Input: part model. Units: mm. Frame: model coordinates. Face numbers are marked on the shaded views. A direction names the side the tool comes from. Coordinates: 2 decimals unless noted, no trailing zeros. Write each loop counter-clockwise with the first axis right and the second up, starting at its lowest first coordinate (ties: lowest second). Pieces come first, ordered by that corner, then holes. Notation, with made-up numbers: (6, 48) - (53, 48) arc R32 ccw to (53, 74) - close; hole circle Ø7 at (28.5, 57.25). An arc over 180 degrees is marked (long way). Use a Markdown table: item, result. Add a question column.
Q1. Section query D-D (z = 16.75). Return the cut outline in (x, y), then the cut area to 3 significant figures.
Q2. Pin query (flat end, axial travel): P1, Ø6, axis at x = 5, z = 15, coming from the +Y side; P2, Ø10, axis at x = -6, z = 12.5, coming from the +Y side; P3, Ø3, axis at y = 2.5, z = 8, coming from the -X side. Return the tip coordinate at first contact, or that it passes through.
Q3. Mould query, pull axis Z, two halves, no side actions, for the marked faces 1, 2, 3 and 4. Classes: released by +Z, released by -Z, zero draft, split by the parting line, or undercut.
Q4. Section query B-B (z = 5). Return the cut outline in (x, y).
Q5. Section query A-A (z = 11). Return the cut outline in (x, y).
Q6. Material intervals for probe 1 along Z at (x, y) = (8.5, 10); probe 2 along X at (y, z) = (-3, 6.5); probe 3 along Y at (x, z) = (2, 12), sorted ascending. Write a range as from..to.
Q7. Section query C-C (z = 2.25). Return the cut outline in (x, y).
Q8. Set-up query: the marked faces 5, 6 and 7. Return all of +Z, -Z, +X, -X, +Y, -Y with unobstructed straight access to the full face (end or side cutting, diameter ignored); none if empty.
from build123d import *

# Parameters (mm, degrees)
ESQUISSE1_W             = 5
ESQUISSE1_H             = 4.088235294
BOSS_EXTRU_1_DEPTH      = 20
ENL_V_START             = -16
ENL_V_MAT_EXTRU_1_DEPTH = 12
CHANFREIN1_SIZE         = 3
ESQUISSE3_R             = 2
ENL_V_MAT_EXTRU_2_DEPTH = 12
ENL_V_START_2           = -8
ESQUISSE4_R             = 4
ENL_V_MAT_EXTRU_3_DEPTH = 12


with BuildPart() as part:
    # Esquisse1 → Boss.-Extru.1 (new body)
    with BuildSketch(Plane.XY):
        with BuildLine():
            ThreePointArc((-14.409025375, 0), (1.090974625, 15.5), (16.590974625, 0))
            Line((16.590974625, 0), (11.590974625, 0))
            Line((11.590974625, 0), (-9.409025375, 0))
            Line((-9.409025375, 0), (-14.409025375, 0))
        make_face()
        with Locations((-11.909025375, -2.044117647)):
            Rectangle(ESQUISSE1_W, ESQUISSE1_H)
        with Locations((14.090974625, -2.044117647)):
            Rectangle(ESQUISSE1_W, ESQUISSE1_H)
    extrude(amount=BOSS_EXTRU_1_DEPTH)

    # Esquisse2 → Enlèv. mat.-Extru.1 (cut)
    with BuildSketch(Plane.XY.offset(20).offset(ENL_V_START)):
        with BuildLine():
            ThreePointArc((-14.409025375, 0), (1.090974625, 11.286497475), (16.590974625, 0))
            ThreePointArc((16.590974625, 0), (1.090974625, 15.5), (-14.409025375, 0))
        make_face()
    extrude(amount=ENL_V_MAT_EXTRU_1_DEPTH, mode=Mode.SUBTRACT)

    # Chanfrein1
    # the kernel refuses this chamfer: 3 mm, written as the material it takes off along each edge
    with BuildSketch(Plane(origin=(1.090974625, 0, 4), x_dir=(0.8782789278300123, -0.4781486431328276, 0), z_dir=(-0.4781486431328276, -0.8782789278300123, 0))) as chanfrein1_piece_1_section:
        Polygon((15.5, -CHANFREIN1_SIZE), (15.5 - CHANFREIN1_SIZE, 0), (15.5, 0), align=None)
    chanfrein1_piece_1 = revolve(axis=Axis((1.090974625, 0, 4), (0, 0, 1)), revolution_arc=237.129113272, mode=Mode.PRIVATE)
    chanfrein1_piece_1 = chanfrein1_piece_1 - Plane(origin=(1.090974625, -5, 2.541086631), x_dir=(-0.9517086177605509, 0.3070027799227584, 0), z_dir=(0, 0, -1)) * Cylinder(16.286497475, 63, mode=Mode.PRIVATE)
    add(chanfrein1_piece_1, mode=Mode.SUBTRACT)
    with BuildSketch(Plane(origin=(1.090974625, 0, 16), x_dir=(0.8782789278300122, -0.4781486431328277, 0), z_dir=(-0.4781486431328277, -0.8782789278300122, 0))) as chanfrein1_piece_2_section:
        Polygon((15.5, CHANFREIN1_SIZE), (15.5 - CHANFREIN1_SIZE, 0), (15.5, 0), align=None)
    chanfrein1_piece_2 = revolve(axis=Axis((1.090974625, 0, 16), (0, 0, 1)), revolution_arc=237.129113272, mode=Mode.PRIVATE)
    chanfrein1_piece_2 = chanfrein1_piece_2 - Plane(origin=(1.090974625, -5, 17.458913369), x_dir=(-0.9517086177605509, 0.3070027799227584, 0), z_dir=(0, 0, -1)) * Cylinder(16.286497475, 62, mode=Mode.PRIVATE)
    add(chanfrein1_piece_2, mode=Mode.SUBTRACT)

    # Esquisse3 → Enlèv. mat.-Extru.2 (cut)
    with BuildSketch(Plane.XZ):
        with Locations(Location((1.090974625, 10, 0), (0, 0, 270))):
            Circle(ESQUISSE3_R)
    extrude(amount=-ENL_V_MAT_EXTRU_2_DEPTH, mode=Mode.SUBTRACT)

    # Esquisse4 → Enlèv. mat.-Extru.3 (cut)
    with BuildSketch(Plane.XZ.offset(ENL_V_START_2)):
        with Locations(Location((1.090974625, 10, 0), (0, 0, 270))):
            Circle(ESQUISSE4_R)
    extrude(amount=-ENL_V_MAT_EXTRU_3_DEPTH, mode=Mode.SUBTRACT)


solid = part.part
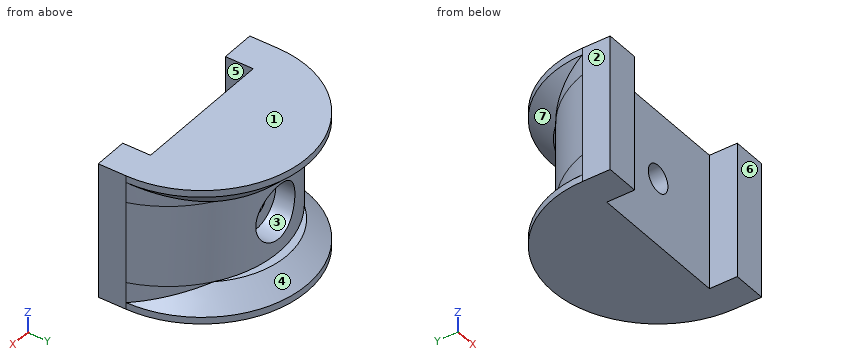
Values follow:
| question | item | result |
|---|---|---|
| 1 | outline | (-14.41, -4.09) - (-9.41, -4.09) - (-9.41, 0) - (11.59, 0) - (11.59, -4.09) - (16.59, -4.09) - (16.59, 0) arc R16.29 ccw to (12.65, 6.47) arc R13.25 ccw to (-10.47, 6.47) arc R16.29 ccw to (-14.41, 0) - close |
| 1 | area | 332 mm2 |
| 2 | P1 | y = 14.06 |
| 2 | P2 | y = 12.6 |
| 2 | P3 | x = -14.05 |
| 3 | face 1 | released by +Z |
| 3 | face 2 | zero draft |
| 3 | face 3 | undercut |
| 3 | face 4 | undercut |
| 4 | outline | (-14.41, -4.09) - (-9.41, -4.09) - (-9.41, 0) - (11.59, 0) - (11.59, -4.09) - (16.59, -4.09) - (16.59, 0) arc R16.29 ccw to (-14.41, 0) - close |
| 5 | outline | (-14.41, -4.09) - (-9.41, -4.09) - (-9.41, 0) - (-0.64, 0) - (-0.64, 8) - (-2.78, 8) - (-2.78, 10.82) arc R16.29 ccw to (-14.41, 0) - close; (2.82, 0) - (11.59, 0) - (11.59, -4.09) - (16.59, -4.09) - (16.59, 0) arc R16.29 ccw to (4.96, 10.82) - (4.96, 8) - (2.82, 8) - close |
| 6 | probe 1 | 0..4, 16..20 |
| 6 | probe 2 | -14.41..-9.41, 11.59..16.59 |
| 6 | probe 3 | 0..8 |
| 7 | outline | (-14.41, -4.09) - (-9.41, -4.09) - (-9.41, 0) - (11.59, 0) - (11.59, -4.09) - (16.59, -4.09) - (16.59, 0) arc R16.29 ccw to (14.85, 3.72) arc R14.25 ccw to (-12.67, 3.72) arc R16.29 ccw to (-14.41, 0) - close |
| 8 | face 5 | +Z, -Z, -Y |
| 8 | face 6 | +Z, -Z, +X, -X, -Y |
| 8 | face 7 | +Y |
